Could you check a few things on this model? Use its own coordinates, in mm. Coordinates: 2 decimals unless noted, no trailing zeros. Loops run counter-clockwise (first coordinate to the right, second up) from the corner with the lowest first, then second, coordinate; pieces in that order, holes last.
1) Imagine slicing it at A-A on z = 29. Please give me the cut outline in (x, y).
2) Will this pin go through, and if not, where does the flat tip stop? P1, Ø1.8, axis at y = -20, z = 29, coming from the +X side.
3) If I drill on line 1 along Y through (x, z) = (-0.55, 29); line 2 along Y through (x, z) = (-0.9, 31.5); line 3 along Y through (x, z) = (-0.9, 31), over which ranges is the centre line in solid material (lowest first)?
4) Imagine slicing it at B-B on y = 20. Please give me the cut outline in (x, z), plus the area to 3 significant figures.
```python
from build123d import *

# Parameters (mm, degrees)
BOSS_EXTRUDE1_DEPTH = 1
SKETCH2_R           = 1.5
CUT_EXTRUDE1_DEPTH  = 10


with BuildPart() as part:
    # Sketch1 → Boss-Extrude1 (new body)
    with BuildSketch(Plane(origin=(0, 0, 0), x_dir=(0, 0, -1), z_dir=(1, 0, 0))):
        with BuildLine():
            Line((-30, 30), (30, 30))
            ThreePointArc((30, 30), (33.535533906, 28.535533906), (35, 25))
            Line((35, 25), (35, -25))
            ThreePointArc((35, -25), (33.535533906, -28.535533906), (30, -30))
            Line((30, -30), (-30, -30))
            ThreePointArc((-30, -30), (-33.535533906, -28.535533906), (-35, -25))
            Line((-35, -25), (-35, 25))
            ThreePointArc((-35, 25), (-33.535533906, 28.535533906), (-30, 30))
        make_face()
    extrude(amount=-BOSS_EXTRUDE1_DEPTH)

    # Sketch2 → Cut-Extrude1 (cut)
    with BuildSketch(Plane(origin=(0, 0, 0), x_dir=(0, 0, -1), z_dir=(1, 0, 0))):
        with Locations((-29, 20)):
            Circle(SKETCH2_R)
        with Locations((-29, -20)):
            Circle(SKETCH2_R)
    extrude(amount=-CUT_EXTRUDE1_DEPTH, mode=Mode.SUBTRACT)


solid = part.part
```
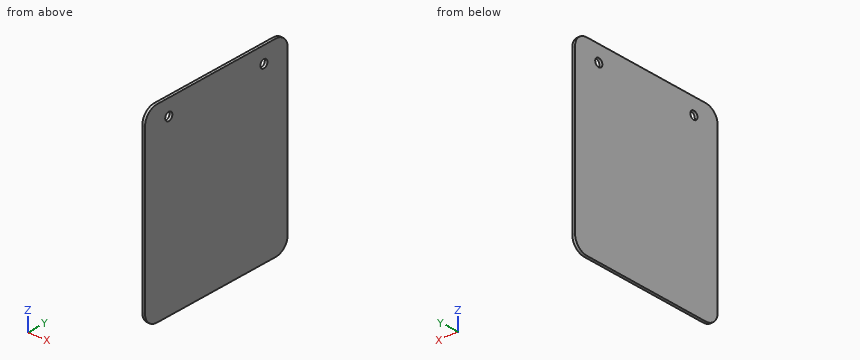
Filled in:
1. outline: (-1, -30) - (0, -30) - (0, -21.5) - (-1, -21.5) - close; (-1, -18.5) - (0, -18.5) - (0, 18.5) - (-1, 18.5) - close; (-1, 21.5) - (0, 21.5) - (0, 30) - (-1, 30) - close
2. P1: passes through
3. line 1: y = -30 to -21.5, -18.5 to 18.5, 21.5 to 30
3. line 2: y = -29.77 to 29.77
3. line 3: y = -29.9 to 29.9
4. outline: (-1, -35) - (0, -35) - (0, 27.5) - (-1, 27.5) - close; (-1, 30.5) - (0, 30.5) - (0, 35) - (-1, 35) - close
4. area: 67.0 mm2
